Here's how the part is built. I have some questions about the finished solid (model axes, mm). Face numbers are marked on the shaded views. A direction names the side the tool comes from. Round coordinates to 2 decimals unless told otherwise and drop trailing zeros. Write each loop counter-clockwise with the first axis right and the second up, starting at its lowest first coordinate (ties: lowest second). Pieces come first, ordered by that corner, then holes. Notation, with made-up numbers: (28.25, 30) -> (42.25, 30) arc R11 ccw to (42.25, 48) -> close; hole circle Ø6 at (29, 1). An arc over 180 degrees is marked (long way). Answer as CSV lines item,"result".
from build123d import *

# Parameters (mm, degrees)
F0_W     = 203.2
F0_H     = 127
F1_DEPTH = 127
F3_DEPTH = 76.2
F4_SIZE2 = 101.6
F4_SIZE  = 76.2
F5_R     = 5.08
F6_R     = 15.24
F7_DEPTH = 50.8
F8_R     = 19.05
F9_DEPTH = 127


with BuildPart() as f1:
    # F0 (on Front) → F1 (new body)
    with BuildSketch(Plane.XZ):
        with Locations((11.5803908557, 1.1079770926)):
            Rectangle(F0_W, F0_H)
    extrude(amount=F1_DEPTH)

    # F2 (on face) → F3 (cut)
    with BuildSketch(Plane.XZ.offset(127)):
        Polygon((-26.5196091443, 1.1079770926), (-26.5196091443, -62.3920229074), (113.1803908557, -62.3920229074), (113.1803908557, 64.6079770926), (11.5803908557, 64.6079770926), (11.5803908557, 1.1079770926), align=None)
    extrude(amount=-F3_DEPTH, mode=Mode.SUBTRACT)

    # F4
    f4_edges = [f1.edges().sort_by_distance(p)[0] for p in [
        (113.180391, -25.4, 64.607977),
    ]]
    f4_side = f1.faces().sort_by_distance((-10.191038, -52.614286, 64.607977))[0]
    chamfer(f4_edges, length=F4_SIZE, length2=F4_SIZE2, reference=f4_side)

    # F5
    f5_edges = [f1.edges().sort_by_distance(p)[0] for p in [
        (11.580391, -88.9, 64.607977),
        (11.580391, -88.9, 1.107977),
        (11.580391, -50.8, 32.857977),
        (-26.519609, -50.8, -30.642023),
        (-26.519609, -127, -30.642023),
        (-26.519609, -88.9, -62.392023),
        (-7.469609, -127, 1.107977),
        (-39.219609, -127, 64.607977),
        (-90.019609, -63.5, 64.607977),
        (-26.519609, 0, 64.607977),
        (-58.269609, -127, -62.392023),
        (-90.019609, -127, 1.107977),
        (43.330391, -50.8, -62.392023),
        (113.180391, -25.4, -62.392023),
        (36.980391, -25.4, 64.607977),
        (113.180391, -25.4, -36.992023),
        (11.580391, 0, -62.392023),
        (-90.019609, 0, 1.107977),
        (-90.019609, -63.5, -62.392023),
        (24.280391, -50.8, 64.607977),
        (-7.469609, -50.8, 1.107977),
    ]]
    fillet(f5_edges, radius=F5_R)

    # F6 (on face) → F7 (cut, through all)
    with BuildSketch(Plane.XZ.offset(50.8)):
        with Locations((29.3603908557, -16.6720229074)):
            Circle(F6_R)
    extrude(amount=-F7_DEPTH, mode=Mode.SUBTRACT)

    # F8 (on face) → F9 (cut)
    with BuildSketch(Plane.XY.offset(64.6079770926)):
        with Locations((-62.1130280197, -75.2307921648)):
            Circle(F8_R)
    extrude(amount=-F9_DEPTH, mode=Mode.SUBTRACT)


solid = f1.part
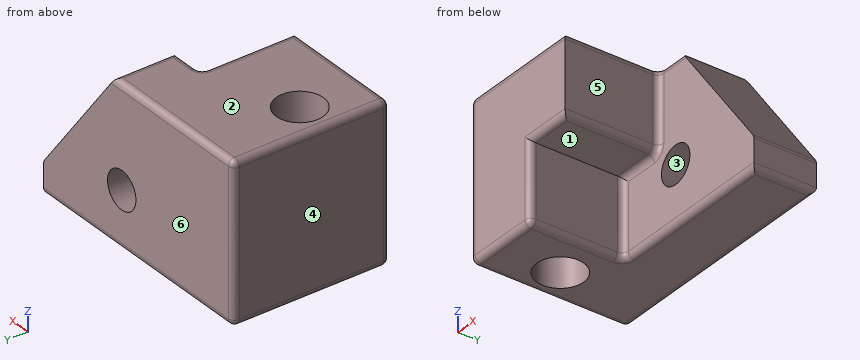
Item 1: Suppose I cut it at B-B, the plane z = 40. List the corners of the cut face in (x, y) for me, then the cut area to 3 significant figures.
Results found:
outline,"(-90.02, -121.92) arc R5.08 ccw to (-84.94, -127) -> (11.58, -127) -> (11.58, -55.88) arc R5.08 cw to (16.66, -50.8) -> (55.44, -50.8) -> (55.44, 0) -> (-84.94, 0) arc R5.08 ccw to (-90.02, -5.08) -> close; hole circle Ø38.1 at (-62.11, -75.23)"
area,"14,000 mm²"
Item 2: For the marked faces 1 and 2, which set-ups out of +Z, -Z, +X, -X, +Y, -Y let a thin tool reach every point of the face, with its end or its side?
Results found:
face 1,"-Z, +X, -Y"
face 2,"+Z, +X, -X, +Y, -Y"
Item 3: Suppose I cut it at C-C, the plane y = -71.5. List the corners of the cut face in (x, z) for me.
Results found:
outline,"(-90.02, -57.31) arc R5.08 ccw to (-84.94, -62.39) -> (-80.79, -62.39) -> (-80.79, 64.61) -> (-84.94, 64.61) arc R5.08 ccw to (-90.02, 59.53) -> close; (-43.43, -62.39) -> (-31.6, -62.39) arc R5.08 ccw to (-26.52, -57.31) -> (-26.52, 1.11) -> (6.5, 1.11) arc R5.08 ccw to (11.58, 6.19) -> (11.58, 59.53) arc R5.08 ccw to (6.5, 64.61) -> (-43.43, 64.61) -> close"
Item 4: Suppose I cut it at D-D, the plane y = -14. List the corners of the cut face in (x, z) for me.
Results found:
outline,"(-90.02, -57.31) arc R5.08 ccw to (-84.94, -62.39) -> (108.1, -62.39) arc R5.08 ccw to (113.18, -57.31) -> (113.18, -38.69) arc R5.08 ccw to (112.16, -35.64) -> (38.5, 62.58) arc R5.08 ccw to (34.44, 64.61) -> (-84.94, 64.61) arc R5.08 ccw to (-90.02, 59.53) -> close; hole circle Ø30.48 at (29.36, -16.67)"
Item 5: Will these pins go through, and if not, where does the flat tip stop? pin 1 (16.5 mm diameter, centred on x = -2, y = -94, fed in from -Z); pin 2 (5 mm diameter, centred on y = -23.5, z = -13.5, fed in from +X); pin 3 (8 mm diameter, centred on y = -29, z = 50, fed in from +X).
Results found:
pin 1,"stops at z = 1.11"
pin 2,"stops at x = 97.44"
pin 3,"stops at x = 50.94"
Item 6: Suppose I cut it at A-A, the plane y = -106. List the corners of the cut face in (x, z) for me.
Results found:
outline,"(-90.02, -57.31) arc R5.08 ccw to (-84.94, -62.39) -> (-31.6, -62.39) arc R5.08 ccw to (-26.52, -57.31) -> (-26.52, 1.11) -> (6.5, 1.11) arc R5.08 ccw to (11.58, 6.19) -> (11.58, 59.53) arc R5.08 ccw to (6.5, 64.61) -> (-84.94, 64.61) arc R5.08 ccw to (-90.02, 59.53) -> close"
Item 7: I need wall thicknesses on L1, parallel to Y at x = 3, z = -27; L2, parallel to Y at x = -51.5, z = -54.5; L3, parallel to X at y = -102, z = 16.5. Which ranges of each line are inside material? Lowest first, please.
Results found:
L1,"y = -50.8 to 0"
L2,"y = -127 to -91.05, -59.41 to 0"
L3,"x = -90.02 to 11.58"
Item 8: If we mould it in two halves opening along X, with no side actions, what happens to the marked faces 3, 4, 5 and 6? For each: pulls with the +X half, pulls with the -X half, needs draft (parallel to the pull), parting line crosses it, or undercut.
Results found:
face 3,"undercut"
face 4,"pulls with the -X half"
face 5,"pulls with the +X half"
face 6,"needs draft"
